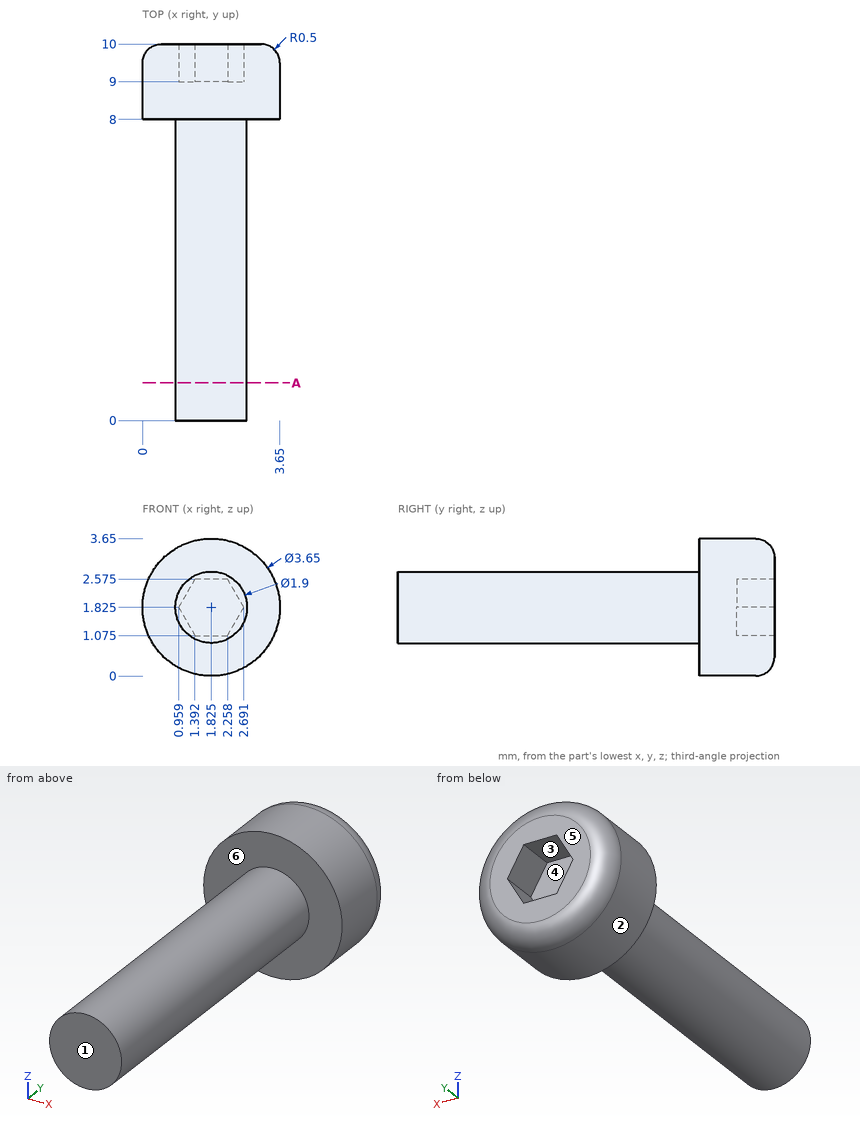
Study the drawing (mm; zero at the part's minimum x, y, z) and answer. A direction names the side the tool comes from. Round coordinates to 2 decimals unless told otherwise and drop trailing zeros. Write each loop counter-clockwise with the first axis right and the second up, starting at its lowest first coordinate (ties: lowest second). Pieces come first, ordered by that corner, then holes. Notation, with made-up numbers: (69.25, -32.5) - (87.25, -32.5) arc R6 cw to (87.25, -23.5) - close; hole circle Ø2 at (-32.75, 35.5). An arc over 180 degrees is marked (long way). Return JSON: item names as keys, results as strings. Group by question number.
Q1. For the marked faces 4, 5 and 6, determine the directions among +Z, -Z, +X, -X, +Y, -Y from which every point of the face is accessible in a straight line to the end or side of a thin tool.
Q2. The mould has two halves that part along Z. Classify the marked faces 1, 2 and 3: released by +Z, released by -Z, zero draft, split by the parting line, or undercut.
Q3. This flat-tipped pin is pushed along its axis until it touches: pin 1 Ø2 at (y, z) = (4.5, 1.5) entering from +X (3 decimals). Where does it stop, or does it pass through?
Q4. Find the intervals of material crossed by L1, parallel to Y at x = 0.75, z = 2.6; L2, parallel to Y at x = 1.3, z = 1.3; L3, parallel to Z at x = 1.75, y = 3, in increasing order.
Q5. The part is cut by section A-A on y = 1. Write down the section's boundary in (x, z) (3 decimals), then the cut area to 3 significant figures.
Solved:
{
 "1": {"face 4": "+Y", "face 5": "+Z, -Z, +X, -X, +Y", "face 6": "-Y"},
 "2": {"face 1": "zero draft", "face 2": "split by the parting line", "face 3": "undercut"},
 "3": {"pin 1": "x = 2.775"},
 "4": {"L1": "8 to 10", "L2": "0 to 9", "L3": "0.88 to 2.77"},
 "5": {"outline": "circle Ø1.9 at (1.825, 1.825)", "area": "2.84 mm²"}
}
